Design review of the part shown in the three views and the two pictorial views. Dimensions are in mm from the part's minimum x, y and z. Give positions to 0.01 mm unless a question says otherwise; leave off trailing zeros. Write each loop counter-clockwise with the first axis right and the second up, starting at its lowest first coordinate (ties: lowest second). Pieces come first, ordered by that corner, then holes.
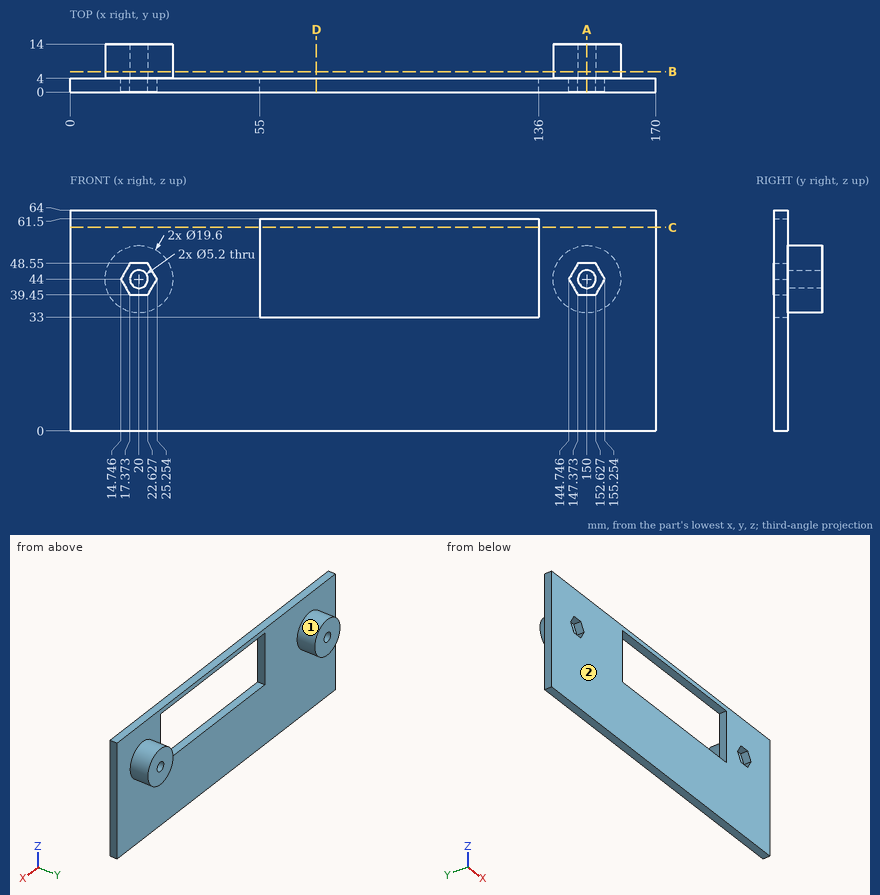
(1) Consider section A-A, the plane x = 150. Give the boundary of the cut face in (y, z), then the cut area to 3 significant figures.
Resolved:
outline: (0, 0) - (4, 0) - (4, 34.2) - (14, 34.2) - (14, 41.4) - (4, 41.4) - (4, 39.45) - (0, 39.45) - close; (0, 48.55) - (4, 48.55) - (4, 46.6) - (14, 46.6) - (14, 53.8) - (4, 53.8) - (4, 64) - (0, 64) - close
area: 364 mm2
(2) Consider section D-D, the plane x = 71.5. Give the boundary of the cut face in (y, z), then the cut area to 3 significant figures.
Resolved:
outline: (0, 0) - (4, 0) - (4, 33) - (0, 33) - close; (0, 61.5) - (4, 61.5) - (4, 64) - (0, 64) - close
area: 142 mm2
(3) Mouldability with a two-part tool opening along X and no side actions: class the marked faces 1 and 2 as pulls with the +X half, pulls with the -X half, needs draft (parallel to the pull), parting line crosses it, or undercut.
Resolved:
face 1: undercut
face 2: needs draft
(4) To check wall thickness, follow L1, parallel to X at y = 6.25, z = 44; L2, parallel to Z at x = 105, y = 2.25; L3, parallel to X at y = 3.75, z = 55. State the ranges of each line that lie inside material, in increasing order.
Resolved:
L1: x = 10.2 to 17.4, 22.6 to 29.8, 140.2 to 147.4, 152.6 to 159.8
L2: z = 0 to 33, 61.5 to 64
L3: x = 0 to 55, 136 to 170
(5) Clearance check with flat-ended pins moving along their axes: P1, Ø4.5, axis at x = 115, y = 2, coming from the -Z side; P2, Ø1.5, axis at x = 34.5, z = 28, coming from the +Y side; P3, Ø8.5, axis at x = 150, z = 44, coming from the -Y side; P4, Ø4.5, axis at x = 20, z = 44, coming from the +Y side. State where each tip first meets the part, or that it passes through.
Resolved:
P1: stops at z = 0
P2: stops at y = 4
P3: stops at y = 4
P4: passes through
(6) Consider section C-C, the plane z = 59. Give the boundary of the cut face in (x, y), then the cut area to 3 significant figures.
Resolved:
outline: (0, 0) - (55, 0) - (55, 4) - (0, 4) - close; (136, 0) - (170, 0) - (170, 4) - (136, 4) - close
area: 356 mm2
(7) Consider section B-B, the plane y = 6. Give the boundary of the cut face in (x, z).
Resolved:
outline: circle Ø19.6 at (20, 44); circle Ø19.6 at (150, 44); hole circle Ø5.2 at (20, 44); hole circle Ø5.2 at (150, 44)
